Can you work these out from the model? Positions are in its coordinate system, mm. Round coordinates to 2 decimals unless told otherwise and drop trailing zeros. Order: outer loops, then holes, each group sorted by start corner. A loop starts at its lowest first (then second) coordinate and runs counter-clockwise, first axis right, second up. Notation, with made-up numbers: M -19,26.25 L 3,26.25 A28 cw 3,50.25 Z; hole C -40,1.25 d2. An arc over 180 degrees is marked long. One line per question, with ' | ' between items.
Autodesk Inventor part; units mm, degrees
ref_plane "YZ Plane" through (0, 0, 0) normal (1, 0, 0) x (0, 1, 0)
ref_plane "XZ Plane" through (0, 0, 0) normal (0, 1, 0) x (-1, 0, 0)
ref_plane "XY Plane" through (0, 0, 0) normal (0, 0, 1) x (1, 0, 0)
sketch "Sketch1" plane through (0, 0, 0) normal (1, 0, 0) x (0, 1, 0)
  line L0 (30.48, -20.9755) -> (30.48, 20.9755)
  line L1 (-30.48, 20.9755) -> (-30.48, -20.9755)
  arc A0 (30.48, 20.9755) -> (-30.48, 20.9755) centre (0, 0) ccw
  arc A1 (-30.48, -20.9755) -> (30.48, -20.9755) centre (0, 0) ccw
  arc A2 (-30.48, -46.9784) -> (-30.48, 46.9784) centre (0, 0) ccw
  arc A3 (-60.48, 32.902) -> (-30.48, 46.9784) centre (-96.5998, 148.8879) ccw
  arc A4 (-30.48, -46.9784) -> (-60.48, -31.098) centre (-134.7727, -207.7233) ccw
  line L2 (56, 0) -> (0, 0) construction
  line L3 (0, 0) -> (-28, 48.4974) construction
  line L4 (0, 0) -> (-28, -48.4974) construction
  line L5 (30.48, 0) -> (56, 0) construction
  line L6 (-18.5, -32.0429) -> (-28, -48.4974) construction
  line L7 (-28, 48.4974) -> (-18.5, 32.0429) construction
  circle A5 centre (43.24, 0) radius 4.5
  circle A6 centre (-23.25, -40.2702) radius 4.5
  circle A7 centre (-23.25, 40.2702) radius 4.5
  line L8 (-60.48, 4.85) -> (-55.98, 4.85)
  line L9 (-55.98, 4.85) -> (-55.98, 6.9)
  line L10 (-55.98, 6.9) -> (-52.98, 6.9)
  line L11 (-52.98, 6.9) -> (-52.98, -6.9)
  line L12 (-52.98, -6.9) -> (-55.98, -6.9)
  line L13 (-55.98, -6.9) -> (-55.98, -4.85)
  line L14 (-55.98, -4.85) -> (-60.48, -4.85)
  line L15 (-60.48, 32.902) -> (-60.48, 4.85)
  line L16 (-60.48, -4.85) -> (-60.48, -31.098)
  point P0 (-72.3678, 0)
  point P1 (-30.48, 0)
  point P2 (-52.98, 0)
  dimension "d1" = 60.96
  dimension "d2" = 30.48
  dimension "d3" = 37
  dimension "d4" = 37
  dimension "d5" = 19
  dimension "d6" = 64
  dimension "d7" = 120
  dimension "d8" = 120
  dimension "d9" = 9
  dimension "d10" = 9
  dimension "d11" = 9
  dimension "d14" = 9.7
  dimension "d15" = 13.8
  dimension "d16" = 4.85
  dimension "d17" = 7.5
  dimension "d18" = 4.5
  dimension "d19" = 30
  dimension "d20" = 30
extrude "Extrusion1" add sketch "Sketch1" along normal blind 3
properties part number "inner"
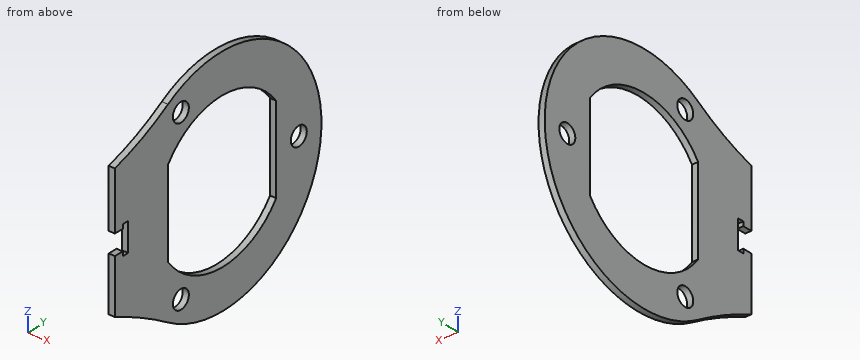
(1) If we section it at C-C on x = 2.35: Please give me the cut outline in (y, z).
Final values:
outline: M -60.48,-31.1 A191.62 cw -30.48,-46.98 A56 ccw long -30.48,46.98 A121.48 cw -60.48,32.9 L -60.48,4.85 L -55.98,4.85 L -55.98,6.9 L -52.98,6.9 L -52.98,-6.9 L -55.98,-6.9 L -55.98,-4.85 L -60.48,-4.85 Z; hole M -30.48,-20.98 A37 ccw 30.48,-20.98 L 30.48,20.98 A37 ccw -30.48,20.98 Z; hole C -23.25,-40.27 d9; hole C -23.25,40.27 d9; hole C 43.24,0 d9
(2) If we section it at B-B on y = 0: Please give me the cut outline in (x, z), plus the area to 3 significant figures.
Final values:
outline: M 0,-56 L 3,-56 L 3,-37 L 0,-37 Z; M 0,37 L 3,37 L 3,56 L 0,56 Z | area: 114 mm^2
(3) Please list where these lines run through material, in increasing order: probe 1 along Y at (x, z) = (1.4, -0.5); probe 2 along Y at (x, z) = (0.4, -2.5); probe 3 along Z at (x, y) = (2.45, -23.25). Write a range as [from, to].
Final values:
probe 1: [-52.98, -30.48], [30.48, 38.77], [47.71, 56] | probe 2: [-52.98, -30.48], [30.48, 39.5], [46.98, 55.94] | probe 3: [-50.95, -44.77], [-35.77, -28.78], [28.78, 35.77], [44.77, 50.95]
(4) Will these pins go through, and if not, where does the flat tip stop? pin 1 Ø1.6 at (x, z) = (1.5, -6) entering from +Y; pin 2 Ø0.9 at (x, y) = (1, -58.5) entering from -Z; pin 3 Ø1.6 at (x, z) = (1, 6.5) entering from +Y.
Final values:
pin 1: y = 55.76 | pin 2: z = -32.14 | pin 3: y = 55.71
(5) If we section it at D-D on y = -23.25: Please give me the cut outline in (x, z), plus the area to 3 significant figures.
Final values:
outline: M 0,-50.95 L 3,-50.95 L 3,-44.77 L 0,-44.77 Z; M 0,-35.77 L 3,-35.77 L 3,-28.78 L 0,-28.78 Z; M 0,28.78 L 3,28.78 L 3,35.77 L 0,35.77 Z; M 0,44.77 L 3,44.77 L 3,50.95 L 0,50.95 Z | area: 79.0 mm^2
(6) If we section it at A-A on z = 0: Please give me the cut outline in (x, y).
Final values:
outline: M 0,-52.98 L 3,-52.98 L 3,-30.48 L 0,-30.48 Z; M 0,30.48 L 3,30.48 L 3,38.74 L 0,38.74 Z; M 0,47.74 L 3,47.74 L 3,56 L 0,56 Z
